Work out the finished part from the listing and answer in its coordinate system (mm). A direction names the side the tool comes from. Round coordinates to 2 decimals unless told otherwise and drop trailing zeros. Loops run counter-clockwise (first coordinate to the right, second up) from the corner with the lowest first, then second, coordinate; pieces in that order, holes last. Notation, with made-up numbers: (41.25, -20) - (98.25, -20) arc R20 ccw to (98.25, 3) - close; hole circle Ø3 at (35.5, -38.75). An arc over 180 degrees is marked (long way). Return JSON: item names as keys, results as strings.
from build123d import *

# Parameters (mm, degrees)
SKETCH152_R     = 1.7
PAD084_DEPTH    = 3
CHAMFER055_SIZE = 1
SKETCH225_R     = 1.6
POCKET053_DEPTH = 3.001


with BuildPart() as part:
    # Sketch152 → Pad084 (new body)
    with BuildSketch(Plane.XY):
        Polygon((40, -30), (-40, -30), (-40, 30), (-30, 30), (-30, 40), (30, 40), (30, 30), (40, 30), align=None)
        with Locations((0, 35)):
            Circle(SKETCH152_R, mode=Mode.SUBTRACT)
        with Locations((-35, 0)):
            Circle(SKETCH152_R, mode=Mode.SUBTRACT)
        with Locations((35, 0)):
            Circle(SKETCH152_R, mode=Mode.SUBTRACT)
    extrude(amount=PAD084_DEPTH)

    # Chamfer055
    chamfer055_edges = [part.edges().sort_by_distance(p)[0] for p in [
        (40, 30, 1.5),
        (30, 40, 1.5),
        (-30, 40, 1.5),
        (-40, 30, 1.5),
        (-40, -30, 1.5),
        (40, -30, 1.5),
    ]]
    chamfer(chamfer055_edges, length=CHAMFER055_SIZE)


with BuildPart() as part_1:
    # Body072 placement: moved
    add(part.part.moved(Location((0, 34.999969, 320.000031))))

    # Sketch225 (on Face2 of Clone003) → Pocket053 (cut, through all)
    with BuildSketch(Plane(origin=(0, 34.999969, 320.000031), x_dir=(1, 0, 0), z_dir=(0, 0, -1))):
        with Locations((-20, 0)):
            Circle(SKETCH225_R)
        with Locations((20, 0)):
            Circle(SKETCH225_R)
        with BuildLine():
            ThreePointArc((-12, 20), (-14.12132, 19.12132), (-15, 17))
            Line((-15, -17), (-15, 17))
            ThreePointArc((-15, -17), (-14.12132, -19.12132), (-12, -20))
            Line((12, -20), (-12, -20))
            ThreePointArc((12, -20), (14.12132, -19.12132), (15, -17))
            Line((15, 17), (15, -17))
            ThreePointArc((15, 17), (14.12132, 19.12132), (12, 20))
            Line((-12, 20), (12, 20))
        make_face()
    extrude(amount=-POCKET053_DEPTH, mode=Mode.SUBTRACT)


solid = part_1.part
1) A tool of negligible diameter and unlimited length cuts with its end or side. For faces 1 (the flat face through (34, 65, 321)), 2 (the cylindrical face through (14.1, 54.14, 321.48)), 3 (the flat face through (1, 56, 323)), from which of +Z, -Z, +X, -X, +Y, -Y can it reach the whole face along a straight path? Write none if from no direction.
Verdict:
{"face 1": "+Z, -Z, +X, +Y", "face 2": "+Z, -Z", "face 3": "+Z, +X, -X, +Y, -Y"}
2) Section C-C (z = 321.5) is taken. Give the vertices of the cut face in (x, y), and give its area (3 significant figures).
Verdict:
{"outline": "(-40, 6) - (-39, 5) - (39, 5) - (40, 6) - (40, 64) - (39, 65) - (30, 65) - (30, 74) - (29, 75) - (-29, 75) - (-30, 74) - (-30, 65) - (-39, 65) - (-40, 64) - close; hole circle Ø3.4 at (-35, 35); hole circle Ø3.2 at (-20, 35); hole (-15, 18) arc R3 ccw to (-12, 15) - (12, 15) arc R3 ccw to (15, 18) - (15, 52) arc R3 ccw to (12, 55) - (-12, 55) arc R3 ccw to (-15, 52) - close; hole circle Ø3.4 at (0, 70); hole circle Ø3.2 at (20, 35); hole circle Ø3.4 at (35, 35)", "area": "4,160 mm2"}
3) Section D-D (x = 0) is taken. Give the vertices of the cut face in (y, z), and give its area (3 significant figures).
Verdict:
{"outline": "(5, 320) - (15, 320) - (15, 323) - (5, 323) - close; (55, 320) - (68.3, 320) - (68.3, 323) - (55, 323) - close; (71.7, 320) - (75, 320) - (75, 323) - (71.7, 323) - close", "area": "79.8 mm2"}
4) Section B-B (x = -35) is taken. Give the vertices of the cut face in (y, z), and give its area (3 significant figures).
Verdict:
{"outline": "(5, 320) - (33.3, 320) - (33.3, 323) - (5, 323) - close; (36.7, 320) - (65, 320) - (65, 323) - (36.7, 323) - close", "area": "170 mm2"}
5) Flat-ended cylindrical pins translate along their axes: pin 1 (2 mm diameter, centred on x = 0, y = 70, fed in from -Z); pin 2 (1.5 mm diameter, centred on x = 32.5, z = 321.5, fed in from +Y); pin 3 (0.9 mm diameter, centred on y = 71.5, z = 322, fed in from +X); pin 4 (1.5 mm diameter, centred on y = 68, z = 321.5, fed in from -X). Find the tip coordinate at first contact, or state that the pin passes through.
Verdict:
{"pin 1": "passes through", "pin 2": "stops at y = 65", "pin 3": "stops at x = 30", "pin 4": "stops at x = -30"}
6) Section A-A (y = 22.5) is taken. Give the vertices of the cut face in (x, z).
Verdict:
{"outline": "(-40, 320) - (-15, 320) - (-15, 323) - (-40, 323) - close; (15, 320) - (40, 320) - (40, 323) - (15, 323) - close"}
7) Find the intervals of material crossed by L1, parallel to Y at x = 0, z = 321.95; L2, parallel to X at y = 26, z = 320.4; L3, parallel to Y at x = -35, z = 322.45, in increasing order.
Verdict:
{"L1": "y = 5 to 15, 55 to 68.3, 71.7 to 75", "L2": "x = -40 to -15, 15 to 40", "L3": "y = 5 to 33.3, 36.7 to 65"}
8) Determine the mould class of faces 4 (the flat face through (0, 75, 321)), 5 (the flat face through (30, 70, 321)), 6 (the flat face through (-30, 69, 321)), 7 (the flat face through (-15, 35, 321)) for opening direction X: pulls with the +X half, pulls with the -X half, needs draft (parallel to the pull), parting line crosses it, or undercut.
Verdict:
{"face 4": "needs draft", "face 5": "pulls with the +X half", "face 6": "pulls with the -X half", "face 7": "undercut"}
